Input: part model. Units: mm. Frame: model coordinates. A direction names the side the tool comes from. Round coordinates to 2 decimals unless told otherwise and drop trailing zeros. Loops run counter-clockwise (first coordinate to the right, second up) from the corner with the lowest first, then second, coordinate; pieces in that order, holes last. Notation, with made-up numbers: (80.25, 84.25) - (105.25, 84.25) arc R28 cw to (105.25, 103.25) - close; hole circle Ø11 at (70, 0.25). An arc over 180 degrees is marked (long way). Write each question's results on one line, items separated by ' | '.
from build123d import *

# Parameters (mm, degrees)
F0_W     = 0.508
F0_H     = 25.908
F1_DEPTH = 431.8
F2_W     = 0.508
F2_H     = 431.8
F3_DEPTH = 25.4
F4_R     = 3.175
F5_DEPTH = 25.4
F6_R     = 3.96875
F6_R_2   = 3.175
F7_DEPTH = 25.4


with BuildPart() as f1:
    # F0 (on Top) → F1 (new body)
    with BuildSketch(Plane.XY):
        with Locations((0.254, -12.954)):
            Rectangle(F0_W, F0_H)
    extrude(amount=F1_DEPTH)

    # F2 (on face) → F3 (join)
    with BuildSketch(Plane.YZ.offset(0.508)):
        with Locations((-25.654, 215.9)):
            Rectangle(F2_W, F2_H)
    extrude(amount=F3_DEPTH)

    # F4 (on face) → F5 (cut)
    with BuildSketch(Plane.YZ.offset(0.508)):
        with Locations((-12.7, 425.45)):
            Circle(F4_R)
        with Locations((-12.7, 29.21)):
            Circle(F4_R)
        with Locations((-12.7, 8.89)):
            Circle(F4_R)
    extrude(amount=-F5_DEPTH, mode=Mode.SUBTRACT)

    # F6 (on face) → F7 (cut)
    with BuildSketch(Plane(origin=(0, -25.4, 0), x_dir=(-1, 0, 0), z_dir=(0, 1, 0))):
        with Locations((-19.558, 400.05)):
            Circle(F6_R)
        with Locations((-13.208, 265.1125)):
            Circle(F6_R_2)
        with Locations((-13.208, 242.8875)):
            Circle(F6_R_2)
        with Locations((-13.208, 19.05)):
            Circle(F6_R_2)
    extrude(amount=-F7_DEPTH, mode=Mode.SUBTRACT)


solid = f1.part
1. Line query: line 1 (Z direction, x = 0.35, y = -12.7) (3 decimals); line 2 (Y direction, x = 12, z = 191.5); line 3 (X direction, y = -12.75, z = 332). Output: solid intervals per line, ascending. Write a range as [from, to].
Answer:
line 1: [0, 5.715], [12.065, 26.035], [32.385, 422.275], [428.625, 431.8] | line 2: [-25.91, -25.4] | line 3: [0, 0.51]
2. Section query A-A, the plane z = 400.05. Output: boundary loops of the cut face in (x, y), plus the area to 3 significant figures.
Answer:
outline: (0, -25.91) - (15.59, -25.91) - (15.59, -25.4) - (0.51, -25.4) - (0.51, 0) - (0, 0) - close; (23.53, -25.91) - (25.91, -25.91) - (25.91, -25.4) - (23.53, -25.4) - close | area: 22.0 mm^2
3. Set-up query: faces 1 (the flat face through (0.508, -13, 213)), 2 (the flat face through (0, -13, 213)). Return all of +Z, -Z, +X, -X, +Y, -Y with unobstructed straight access to the full face (end or side cutting, diameter ignored); none if empty.
Answer:
face 1: +Z, -Z, +X, +Y | face 2: +Z, -Z, -X, +Y, -Y
4. Section query B-B, the plane z = 278.5. Output: boundary loops of the cut face in (x, y), plus the area to 3 significant figures.
Answer:
outline: (0, -25.91) - (25.91, -25.91) - (25.91, -25.4) - (0.51, -25.4) - (0.51, 0) - (0, 0) - close | area: 26.1 mm^2
5. Contact query for flat-ended pins moving along their axis: pin 1 (2 mm diameter, centred on y = -11, z = 312, fed in from +X); pin 2 (8 mm diameter, centred on x = 17, z = 331, fed in from +Y); pin 3 (7 mm diameter, centred on x = 19.558, z = 400.05, fed in from +Y). Output: stop coordinate, or through.
Answer:
pin 1: x = 0.51 | pin 2: y = -25.4 | pin 3: through
6. Mould query, pull axis Z, two halves, no side actions, for faces 3 (the cylindrical face through (20.075, -25.65, 403.985)), 4 (the flat face through (13, -25.4, 213)). Classes: pulls with the +Z half, pulls with the -Z half, needs draft (parallel to the pull), parting line crosses it, or undercut.
Answer:
face 3: undercut | face 4: needs draft
